```python
from build123d import *

# Parameters (mm, degrees)
SKETCH_1_W                  = 55
SKETCH_1_H                  = 60
EXTRUDE_1_DEPTH             = 16.5
HOLE_WIZARD_3_6_3_6_1_D     = 3.6
HOLE_WIZARD_3_6_3_6_1_DEPTH = 25
HOLE_WIZARD_3_6_3_6_1_TIP   = 1.081549114
HOLE_WIZARD_M2_5_1_D        = 2.05
HOLE_WIZARD_M2_5_1_DEPTH    = 14
HOLE_WIZARD_M2_5_1_TIP      = 0.615882135
SKETCH_8_W                  = 35
SKETCH_8_H                  = 20.4
CUT_EXTRUDE_1_DEPTH         = 44.914690025
CUT_EXTRUDE_START           = 2.5
SKETCH_9_W                  = 20
SKETCH_9_H                  = 6
CUT_EXTRUDE_2_DEPTH         = 42.414690025
SHELL_START                 = 1.8
SHELL_1_DEPTH               = 14.7
EXTRUDE_2_DEPTH             = 4
SKETCH_16_R                 = 3
CUT_EXTRUDE_4_DEPTH         = 12
CUT_EXTRUDE_5_DEPTH         = 45.787721532
CUT_EXTRUDE_5_DEPTH_BACK    = 45.787721532
SKETCH_17_R                 = 2.5
FILLET_1_R                  = 0.5
FILLET_2_R                  = 0.5
SKETCH_21_W                 = 70
SKETCH_21_H                 = 90
EXTRUDE_3_DEPTH             = 4
SKETCH_24_R                 = 8.656208536
SKETCH_24_R_2               = 4.782814597
EXTRUDE_4_DEPTH             = 4
HOLE_WIZARD_6_5_6_5_1_D     = 6.5
HOLE_WIZARD_1_D             = 6.6
HOLE_WIZARD_1_DEPTH         = 17
HOLE_WIZARD_1_CSINK_D       = 13.2
HOLE_WIZARD_1_CSINK_ANGLE   = 90
HOLE_WIZARD_1_TIP           = 1.982840043
FILLET_3_R                  = 3


# Read off the part's stored shape, not the designer's step: 抽壳1
with BuildPart() as part:
    # 草图1 → 凸台-拉伸1 (new body)
    with BuildSketch(Plane.XY):
        Rectangle(SKETCH_1_W, SKETCH_1_H)
    extrude(amount=EXTRUDE_1_DEPTH)

    # Ø3.6 (3.6) 直径孔1
    with Locations(Plane.XY.offset(16.5)):
        with Locations((-24, 21.5), (24, 21.5), (24, -6), (-15, -26.5)):
            Hole(HOLE_WIZARD_3_6_3_6_1_D / 2, depth=HOLE_WIZARD_3_6_3_6_1_DEPTH)
            with Locations((0, 0, -(HOLE_WIZARD_3_6_3_6_1_DEPTH + HOLE_WIZARD_3_6_3_6_1_TIP / 2))):  # 118° drill point
                Cone(0, HOLE_WIZARD_3_6_3_6_1_D / 2, HOLE_WIZARD_3_6_3_6_1_TIP, mode=Mode.SUBTRACT)

    # M2.5 螺纹孔1
    with Locations(Plane.XY.offset(16.5)):
        with Locations((-24, 26.5), (24, 26.5), (24, -1), (-22.5, -26.5)):
            Hole(HOLE_WIZARD_M2_5_1_D / 2, depth=HOLE_WIZARD_M2_5_1_DEPTH)
            with Locations((0, 0, -(HOLE_WIZARD_M2_5_1_DEPTH + HOLE_WIZARD_M2_5_1_TIP / 2))):  # 118° drill point
                Cone(0, HOLE_WIZARD_M2_5_1_D / 2, HOLE_WIZARD_M2_5_1_TIP, mode=Mode.SUBTRACT)

    # 草图8 → 切除-拉伸1 (cut, through all)
    with BuildSketch(Plane.XY.offset(16.5)):
        with Locations((10, -19.8)):
            Rectangle(SKETCH_8_W, SKETCH_8_H)
    extrude(amount=-CUT_EXTRUDE_1_DEPTH, mode=Mode.SUBTRACT)

    # 草图9 → 切除-拉伸2 (cut, through all)
    with BuildSketch(Plane(origin=(0, 0, 16.5), x_dir=(-1, 0, 0), z_dir=(0, 0, -1)).offset(CUT_EXTRUDE_START)):
        with Locations((17.5, -27)):
            Rectangle(SKETCH_9_W, SKETCH_9_H)
    extrude(amount=CUT_EXTRUDE_2_DEPTH, mode=Mode.SUBTRACT)

    # 抽壳1 outline → 抽壳1 (cut)
    with BuildSketch(Plane.XY.offset(SHELL_START)):
        with BuildLine():
            ThreePointArc((-21.743758657, 28.2), (-21.182110509, 26.299690696), (-22.006919283, 24.4979375))
            ThreePointArc((-22.006919283, 24.4979375), (-20.910890356, 19.651378458), (-25.7, 18.326673669))
            Line((-25.7, 18.326673669), (-25.7, -22.2))
            Line((-25.7, -22.2), (-9.3, -22.2))
            Line((-9.3, -22.2), (-9.3, -7.8))
            Line((-9.3, -7.8), (20.882308546, -7.8))
            ThreePointArc((20.882308546, -7.8), (20.494996561, -5.178446051), (22.006919283, -3.0020625))
            ThreePointArc((22.006919283, -3.0020625), (21.865811165, 0.8509087), (25.7, 1.256241343))
            Line((25.7, 1.256241343), (25.7, 18.326673669))
            ThreePointArc((25.7, 18.326673669), (20.910890356, 19.651378458), (22.006919283, 24.4979375))
            ThreePointArc((22.006919283, 24.4979375), (21.182110509, 26.299690696), (21.743758657, 28.2))
            Line((21.743758657, 28.2), (-21.743758657, 28.2))
        make_face()
    extrude(amount=SHELL_1_DEPTH, mode=Mode.SUBTRACT)

    # 草图16 → 切除-拉伸4 (cut)
    with BuildSketch(Plane(origin=(-7.5, 0, 0), x_dir=(0, 0, -1), z_dir=(1, 0, 0))):
        with Locations(Location((-8, -18, 0), (0, 0, 90))):
            Circle(SKETCH_16_R)
    extrude(amount=-CUT_EXTRUDE_4_DEPTH, mode=Mode.SUBTRACT)


with BuildPart() as body_2:
    # 草图10 → 凸台-拉伸2 (new body)
    with BuildSketch(Plane.XY.offset(16.5)):
        Polygon((-27.5, -30), (-7.5, -30), (-7.5, -9.6), (27.5, -9.6), (27.5, 30), (-27.5, 30), align=None)
    extrude(amount=EXTRUDE_2_DEPTH)


with BuildPart() as cut_extrude_5_tool:
    # 草图17 → 切除-拉伸5 (new, two sides: drawn at the far end of the back side and taken through both)
    with BuildSketch(Plane.XY.offset(1.8).offset(-CUT_EXTRUDE_5_DEPTH_BACK)):
        with Locations((6.5, 9.5)):
            Circle(SKETCH_17_R)
    extrude(amount=CUT_EXTRUDE_5_DEPTH + CUT_EXTRUDE_5_DEPTH_BACK)


with BuildPart() as part_1:
    add(part.part)

    # 切除-拉伸5: cut by cut_extrude_5_tool
    add(cut_extrude_5_tool.part, mode=Mode.SUBTRACT)

    # 圆角1
    fillet_1_edges = [part_1.edges().sort_by_distance(p)[0] for p in [
        (-27.5, 3, 0),
        (0, 30, 0),
        (27.5, 10.2, 0),
        (27.5, -9.6, 8.25),
        (-7.5, -16.8, 0),
        (10, -9.6, 0),
        (-7.5, -9.6, 8.25),
        (-7.5, -30, 15.25),
        (-27.5, -30, 15.25),
        (-27.5, 30, 8.25),
        (27.5, 30, 8.25),
        (-17.5, -24, 0),
        (-7.5, -24, 7),
        (-27.5, -24, 7),
    ]]
    fillet(fillet_1_edges, radius=FILLET_1_R)


with BuildPart() as body_2_1:
    add(body_2.part)

    # 切除-拉伸5: cut by cut_extrude_5_tool
    add(cut_extrude_5_tool.part, mode=Mode.SUBTRACT)

    # 圆角2
    fillet_2_edges = [body_2_1.edges().sort_by_distance(p)[0] for p in [
        (-27.5, 30, 18.5),
        (27.5, 30, 18.5),
        (27.5, -9.6, 18.5),
        (-7.5, -9.6, 18.5),
        (-7.5, -30, 18.5),
        (-27.5, -30, 18.5),
    ]]
    fillet(fillet_2_edges, radius=FILLET_2_R)

    # 草图21 → 凸台-拉伸3 (add)
    with BuildSketch(Plane.XY.offset(20.5)):
        Rectangle(SKETCH_21_W, SKETCH_21_H)
        with BuildLine():
            Line((-27, -30), (-8, -30))
            ThreePointArc((-8, -30), (-7.646446609, -29.853553391), (-7.5, -29.5))
            Line((-7.5, -29.5), (-7.5, -10.1))
            ThreePointArc((-7.5, -10.1), (-7.353553391, -9.746446609), (-7, -9.6))
            Line((-7, -9.6), (27, -9.6))
            ThreePointArc((27, -9.6), (27.353553391, -9.453553391), (27.5, -9.1))
            Line((27.5, -9.1), (27.5, 29.5))
            ThreePointArc((27.5, 29.5), (27.353553391, 29.853553391), (27, 30))
            Line((27, 30), (-27, 30))
            ThreePointArc((-27, 30), (-27.353553391, 29.853553391), (-27.5, 29.5))
            Line((-27.5, 29.5), (-27.5, -29.5))
            ThreePointArc((-27.5, -29.5), (-27.353553391, -29.853553391), (-27, -30))
        make_face(mode=Mode.SUBTRACT)
    extrude(amount=-EXTRUDE_3_DEPTH)

    # 草图24 → 凸台-拉伸4 (add)
    with BuildSketch(Plane(origin=(0, 0, 16.5), x_dir=(-1, 0, 0), z_dir=(0, 0, -1))):
        with Locations((-6.5, 9.5)):
            Circle(SKETCH_24_R)
        with Locations((-6.5, 9.5)):
            Circle(SKETCH_24_R_2, mode=Mode.SUBTRACT)
    extrude(amount=-EXTRUDE_4_DEPTH)

    # Ø6.5 (6.5) 直径孔1 (through all)
    with Locations(Plane.XY.offset(20.5)):
        with Locations((-28, 36), (28, 36), (28, -36), (-28, -36)):
            Hole(HOLE_WIZARD_6_5_6_5_1_D / 2)

    # 打孔尺寸(%根据十字)槽沉头木螺钉的类型1
    with Locations(Plane.XY.offset(20.5)):
        with Locations((6.5, 9.5)):
            CounterSinkHole(HOLE_WIZARD_1_D / 2, HOLE_WIZARD_1_CSINK_D / 2, depth=HOLE_WIZARD_1_DEPTH, counter_sink_angle=HOLE_WIZARD_1_CSINK_ANGLE)
            with Locations((0, 0, -(HOLE_WIZARD_1_DEPTH + HOLE_WIZARD_1_TIP / 2))):  # 118° drill point
                Cone(0, HOLE_WIZARD_1_D / 2, HOLE_WIZARD_1_TIP, mode=Mode.SUBTRACT)

    # 圆角3
    fillet_3_edges = [body_2_1.edges().sort_by_distance(p)[0] for p in [
        (-35, 45, 18.5),
        (-35, -45, 18.5),
        (35, -45, 18.5),
        (35, 45, 18.5),
    ]]
    fillet(fillet_3_edges, radius=FILLET_3_R)


solid = body_2_1.part
```
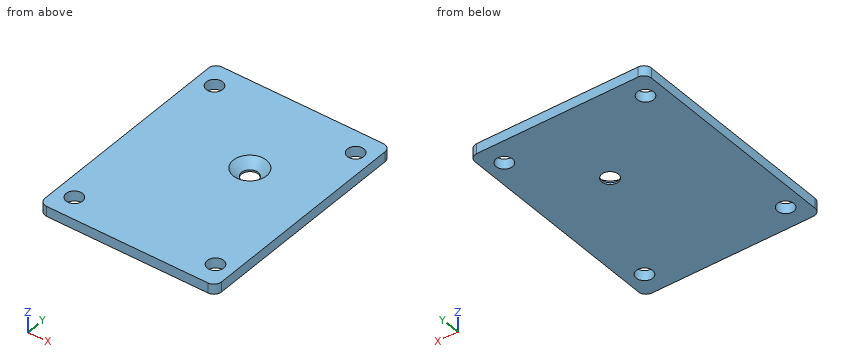
Source: CAD feature listing. Evaluate the final solid. Frame: model axes, mm. Round coordinates to 2 decimals unless told otherwise and drop trailing zeros. Write each loop counter-clockwise with the first axis right and the second up, starting at its lowest first coordinate (ties: lowest second). Pieces come first, ordered by that corner, then holes. Notation, with made-up numbers: M 31,81.25 L 87,81.25 A29 cw 87,119.25 Z; hole C 23.25,87 d11. An arc over 180 degrees is marked long. Answer as a JSON object with one key per item and string values. Group by question number.
(1) Section query C-C on z = 18.35. Output: boundary loops of the cut face in (x, y), then the cut area to 3 significant figures.
(2) Section query B-B on x = 28. Output: boundary loops of the cut face in (y, z), then the cut area to 3 significant figures.
(3) Section query A-A on y = 36. Output: boundary loops of the cut face in (x, z), then the cut area to 3 significant figures.
(4) Ray query, line 1 (Y direction, x = -28, z = 17.8); line 2 (X direction, y = -33.5, z = 18.55); line 3 (X direction, y = 9.5, z = 16.8). Return the intervals inside material, ascending. Write a range as [from, to].
(5) Section query D-D on x = 6.5. Output: boundary loops of the cut face in (y, z), then the cut area to 3 significant figures.
Computed values:
{
 "1": {"outline": "M -35,-42 A3 ccw -32,-45 L 32,-45 A3 ccw 35,-42 L 35,42 A3 ccw 32,45 L -32,45 A3 ccw -35,42 Z; hole C -28,-36 d6.5; hole C -28,36 d6.5; hole C 6.5,9.5 d8.9; hole C 28,-36 d6.5; hole C 28,36 d6.5", "area": "6,100 mm^2"},
 "2": {"outline": "M -45,16.5 L -39.25,16.5 L -39.25,20.5 L -45,20.5 Z; M -32.75,16.5 L 32.75,16.5 L 32.75,20.5 L -32.75,20.5 Z; M 39.25,16.5 L 45,16.5 L 45,20.5 L 39.25,20.5 Z", "area": "308 mm^2"},
 "3": {"outline": "M -35,16.5 L -31.25,16.5 L -31.25,20.5 L -35,20.5 Z; M -24.75,16.5 L 24.75,16.5 L 24.75,20.5 L -24.75,20.5 Z; M 31.25,16.5 L 35,16.5 L 35,20.5 L 31.25,20.5 Z", "area": "228 mm^2"},
 "4": {"line 1": "[-45, -39.25], [-32.75, 32.75], [39.25, 45]", "line 2": "[-35, -30.08], [-25.92, 25.92], [30.08, 35]", "line 3": "[-35, 3.2], [9.8, 35]"},
 "5": {"outline": "M -45,16.5 L 6.2,16.5 L 6.2,17.2 L 2.9,20.5 L -45,20.5 Z; M 12.8,16.5 L 45,16.5 L 45,20.5 L 16.1,20.5 L 12.8,17.2 Z", "area": "323 mm^2"}
}
